The drawing under review shows one solid part. Ordinate dimensions are in mm from its lowest x, y, z. Round coordinates to 2 decimals unless told otherwise and drop trailing zeros. Write each loop counter-clockwise with the first axis right and the second up, starting at its lowest first coordinate (ties: lowest second). Pieces come first, ordered by that corner, then holes. Notation, with made-up numbers: (41, -21) -> (59, -21) arc R22 cw to (59, 17) -> close; hole circle Ø7 at (6.25, 6.25). An arc over 180 degrees is marked (long way). Write item = value, one per line. Start each with the question number.
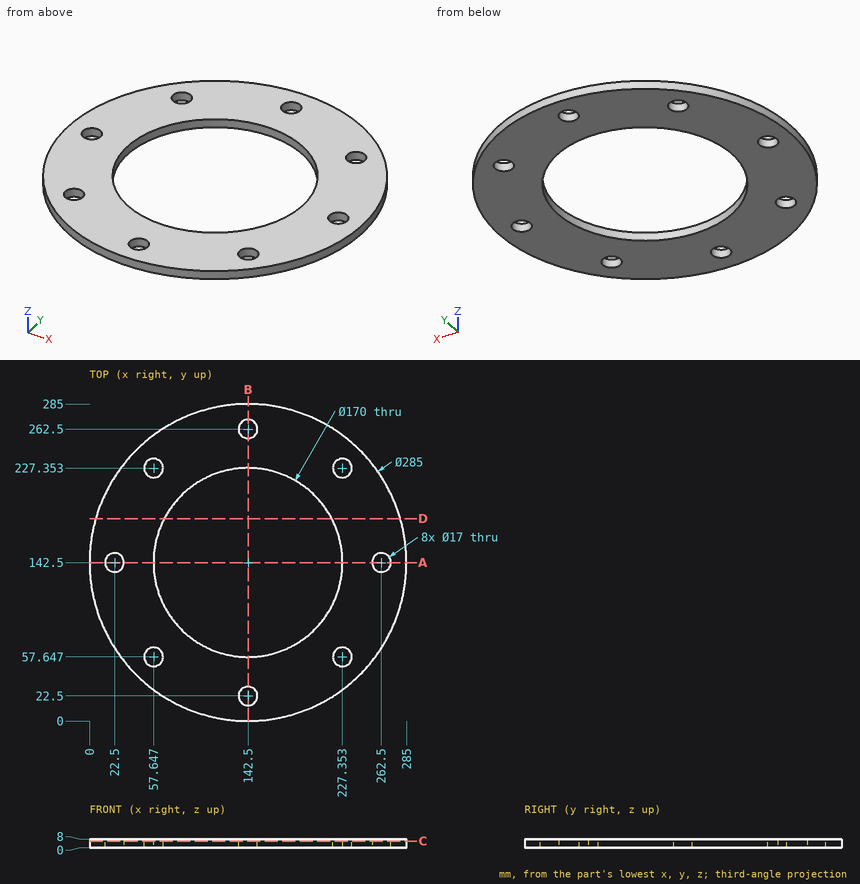
1. Clearance check with flat-ended pins moving along their axes: pin 1 Ø1 at (x, z) = (53, 5) entering from +Y; pin 2 Ø10 at (x, y) = (142.5, 22.5) entering from +Z; pin 3 Ø1 at (x, z) = (55.5, 5.5) entering from -Y; pin 4 Ø3 at (x, z) = (87.5, 1) entering from +Y. State where each tip first meets the part, or that it passes through.
2. Consider section C-C, the plane z = 6. Give the number of separate pieces and of enclosed holes in the cut face, then the cut area to 3 significant figures.
3. Consider section A-A, the plane y = 142.5. Give the boundary of the cut face in (x, z), then the cut area to 3 significant figures.
4. Consider section D-D, the plane y = 182. Give the boundary of the cut face in (x, z).
5. Wall thickness on L1, parallel to X at y = 53.5, z = 5.75; L2, parallel to Y at x = 187, z = 2.25; L3, parallel to X at y = 258, z = 2: over which ranges is each line inside the solid? List them lowest first. Write a range as from..to.
Outcome:
q1.pin_1 = 253.79
q1.pin_2 = through
q1.pin_3 = 29.26
q1.pin_4 = 274.58
q2.separate_pieces = 1
q2.enclosed_holes = 9
q2.area = 39,300 mm2
q3.outline = (0, 0) -> (14, 0) -> (14, 8) -> (0, 8) -> close; (31, 0) -> (57.5, 0) -> (57.5, 8) -> (31, 8) -> close; (227.5, 0) -> (254, 0) -> (254, 8) -> (227.5, 8) -> close; (271, 0) -> (285, 0) -> (285, 8) -> (271, 8) -> close
q3.area = 648 mm2
q4.outline = (5.58, 0) -> (67.24, 0) -> (67.24, 8) -> (5.58, 8) -> close; (217.76, 0) -> (279.42, 0) -> (279.42, 8) -> (217.76, 8) -> close
q5.L1 = 31.21..50.23, 65.07..219.93, 234.77..253.79
q5.L2 = 7.13..70.08, 214.92..277.87
q5.L3 = 59.04..135.29, 149.71..225.96
